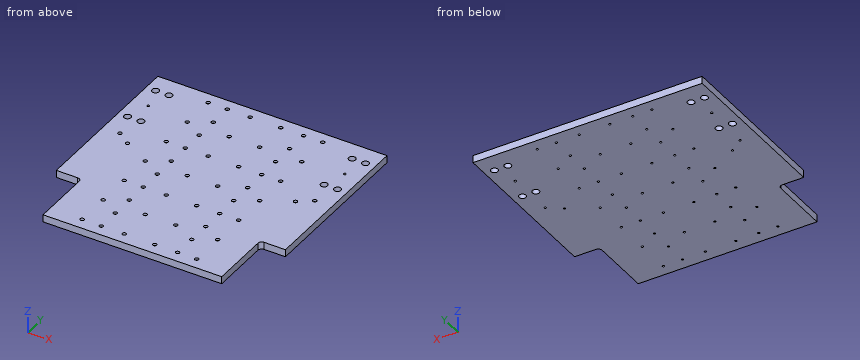
from build123d import *

# Parameters (mm, degrees)
SKETCH1_W                      = 600
SKETCH1_H                      = 600
BOSS_EXTRUDE1_DEPTH            = 19.05
SKETCH2_W                      = 65.95
SKETCH2_H                      = 165
CUT_EXTRUDE1_DEPTH             = 425.69153806
FILLET1_R                      = 10
SKETCH5_R                      = 9.017
SKETCH5_R_2                    = 3.175
CUT_EXTRUDE2_DEPTH             = 425.69153806
CBORE_FOR_M5_SHCS1_D           = 5.5
CBORE_FOR_M5_SHCS1_DEPTH       = 28.347633298
CBORE_FOR_M5_SHCS1_CBORE_D     = 10
CBORE_FOR_M5_SHCS1_CBORE_DEPTH = 6
CBORE_FOR_M5_SHCS1_TIP         = 1.652366702


with BuildPart() as part:
    # Sketch1 → Boss-Extrude1 (new body)
    with BuildSketch(Plane.XY):
        Rectangle(SKETCH1_W, SKETCH1_H)
    extrude(amount=BOSS_EXTRUDE1_DEPTH)

    # Sketch2 → Cut-Extrude1 (cut, through all)
    with BuildSketch(Plane(origin=(0, 0, 0), x_dir=(-1, 0, 0), z_dir=(0, 0, -1))):
        with Locations((267.025, -217.5)):
            Rectangle(SKETCH2_W, SKETCH2_H)
        with Locations((-267.025, -217.5)):
            Rectangle(SKETCH2_W, SKETCH2_H)
    extrude(amount=-CUT_EXTRUDE1_DEPTH, mode=Mode.SUBTRACT)

    # Fillet1
    fillet1_edges = [part.edges().sort_by_distance(p)[0] for p in [
        (-234.05, -135, 9.525),
        (234.05, -135, 9.525),
    ]]
    fillet(fillet1_edges, radius=FILLET1_R)

    # Sketch5 → Cut-Extrude2 (cut, through all)
    with BuildSketch(Plane(origin=(0, 0, 0), x_dir=(-1, 0, 0), z_dir=(0, 0, -1))):
        with Locations((240, 249)):
            Circle(SKETCH5_R)
        with Locations((275, 249)):
            Circle(SKETCH5_R)
        with Locations((257.5, 189)):
            Circle(SKETCH5_R_2)
        with Locations((275, 129)):
            Circle(SKETCH5_R)
        with Locations((240, 129)):
            Circle(SKETCH5_R)
        with Locations((-275, 129)):
            Circle(SKETCH5_R)
        with Locations((-240, 129)):
            Circle(SKETCH5_R)
        with Locations((-257.5, 189)):
            Circle(SKETCH5_R_2)
        with Locations((-275, 249)):
            Circle(SKETCH5_R)
        with Locations((-240, 249)):
            Circle(SKETCH5_R)
    extrude(amount=-CUT_EXTRUDE2_DEPTH, mode=Mode.SUBTRACT)

    # CBORE for M5 SHCS1
    with Locations(Plane.XY.offset(19.05)):
        with Locations((-100, 210), (-100, 270), (100, 270), (100, 210), (100, 150), (-100, 150), (-100, 90), (100, 90), (100, 30), (-100, 30), (-255, 64), (-220, 39), (255, 64), (220, 39), (100, -30), (-100, -30), (-100, -90), (100, -90), (100, -150), (-100, -150), (-100, -210), (100, -210), (100, -270), (-100, -270), (150, -270), (150, -180), (150, -90), (150, 0), (150, 90), (150, 180), (150, 270), (40, 270), (40, 180), (-40, 180), (-40, 270), (-150, 270), (-150, 180), (-150, 90), (-40, 90), (40, 90), (40, 0), (-40, 0), (-40, -90), (40, -90), (-150, -90), (-150, 0), (-150, -180), (-150, -270), (-40, -270), (-40, -180), (40, -180), (40, -270)):
            CounterBoreHole(CBORE_FOR_M5_SHCS1_D / 2, CBORE_FOR_M5_SHCS1_CBORE_D / 2, CBORE_FOR_M5_SHCS1_CBORE_DEPTH, depth=CBORE_FOR_M5_SHCS1_DEPTH)
            with Locations((0, 0, -(CBORE_FOR_M5_SHCS1_DEPTH + CBORE_FOR_M5_SHCS1_TIP / 2))):  # 118° drill point
                Cone(0, CBORE_FOR_M5_SHCS1_D / 2, CBORE_FOR_M5_SHCS1_TIP, mode=Mode.SUBTRACT)


solid = part.part
CAD build for the part. Positions are in the model's coordinates, mm. Round coordinates to 2 decimals unless told otherwise and drop trailing zeros.
(1) Probe line 1 along Y through (x, z) = (255, 4.5); line 2 along Y through (x, z) = (219.5, 5.75); line 3 along Y through (x, z) = (240, 9). List the from-to ranges inside material, lowest first.
(2) Slice it at A-A, the plane z = 6.5. Count the separate pieces of the cut face and the enclosed holes in it, and give its area (3 significant figures).
(3) Drop flat-ended pins along their axis: P1, Ø3, axis at x = -40.5, y = -178, coming from the +Z side; P2, Ø8, axis at x = -150, y = 90, coming from the -Z side. Give the stop position or say it passes through.
From the geometry:
1. line 1: y = -135 to 61.25, 66.75 to 187.04, 190.96 to 300
1. line 2: y = -300 to 36.3, 41.7 to 300
1. line 3: y = -135.86 to 119.98, 138.02 to 239.98, 258.02 to 300
2. separate pieces: 1
2. enclosed holes: 62
2. area: 335,000 mm2
3. P1: stops at z = 13.05
3. P2: stops at z = 0
